Autodesk Inventor part; units mm, degrees
ref_plane "Work Plane3" through (10, 0, 0) normal (1, 0, 0) x (0, 1, 0)
ref_plane "Work Plane5" through (-12.5, 0, 0) normal (1, 0, 0) x (0, 1, 0)
ref_plane "XZ Plane" through (0, 0, 0) normal (0, 1, 0) x (-1, 0, 0)
sketch "Sketch19" plane through (0, 0, 0) normal (0, 0, 1) x (1, 0, 0)
  circle A0 centre (0, 0) radius 12.5
  dimension "d130" = 25
extrude "Extrusion17" add sketch "Sketch19" along normal blind 40
sketch "Sketch20" plane through (0, 0, 40) normal (0, 0, 1) x (1, 0, 0)
  circle A0 centre (0, 0) radius 10
  dimension "d133" = 20
fillet "Fillet6" radius 10 1 edges at (-12.5, 0, 0)
extrude "Extrusion18" cut sketch "Sketch20" against normal blind 36
ref_plane "Work Plane3" through (10, 0, 0) normal (1, 0, 0) x (0, 1, 0)
sketch "Sketch21" plane through (10, 0, 0) normal (1, 0, 0) x (0, 1, 0)
  line L0 (0, 0) -> (0, 20)
  circle A0 centre (0, 20) radius 2.85
  dimension "d138" = 20
  dimension "d139" = 5.7
extrude "Extrusion19" add sketch "Sketch21" along normal blind 14.5
sketch "Sketch26" plane through (0, 0, 0) normal (1, 0, 0) x (0, 1, 0)
  line L0 (-10, 40) -> (10, 40)
  line L1 (12.5, 40) -> (-12.5, 40)
  line L2 (10, 40) -> (12.5, 40)
  line L3 (17.5, 60) -> (12.5, 40)
  line L4 (17.5, 60) -> (17.5, 62.5)
  line L5 (17.5, 62.5) -> (15, 62.5)
  line L6 (15, 62.5) -> (15, 60)
  line L7 (10, 40) -> (15, 60)
  line L8 (0, -10.5) -> (0, 63)
  point P0 (0, 0)
  dimension "d147" = 2.5
  dimension "d148" = 2.5
revolve "Revolution1" add sketch "Sketch26" angle 360 about axis through (0, 0, -10) along (0, 0, 1)
sketch "Sketch27" plane through (0, 0, 0) normal (1, 0, 0) x (0, 1, 0)
  line L0 (12.5, 40) -> (13.7856, 41.5321)
  line L1 (12.5, 40) -> (14.5, 40) construction
  line L2 (13.7856, 41.5321) -> (17.5, 60)
  line L3 (12.5, 40) -> (-12.5, 40)
  line L4 (12.5, 40) -> (11.5, 40)
  line L5 (-17.5, 60) -> (17.5, 60)
  line L6 (17.5, 60) -> (16.5, 60)
  line L7 (16.5, 60) -> (11.5, 40)
  point P0 (0, 0)
  dimension "d150" = 2
  dimension "d151" = 50
  dimension "d152" = 1
  dimension "d153" = 1
extrude "Extrusion21" add sketch "Sketch27" along normal mid plane 2
pattern_circular "Circular Pattern2" count 8 over 360 about axis through (0, 0, -10) along (0, 0, 1) of "Extrusion21"
fillet "Fillet7" radius 5 1 edges at (-10, 0, 4)
ref_plane "Work Plane5" through (-12.5, 0, 0) normal (1, 0, 0) x (0, 1, 0)
sketch "Sketch30" plane through (-12.5, 0, 0) normal (1, 0, 0) x (0, 1, 0)
  circle A0 centre (0, 20) radius 2.85
  line L0 (0, 0) -> (0, 20)
  circle A1 centre (0, 20) radius 3.65
  line L1 (0, 20) -> (0, 35)
  circle A2 centre (0, 35) radius 2.15
  line L2 (0, 20) -> (-3.15, 20)
  line L3 (-3.15, 20) -> (3.15, 20)
  line L4 (2.15, 35) -> (3.15, 20)
  line L5 (-3.15, 20) -> (-2.1453, 35.1423)
  point P0 (2.9808, 20.3389)
  point P1 (-2.9809, 20.3376)
  point P2 (3.0126, 22.0607)
  point P3 (-3.0133, 22.0597)
  dimension "d166" = 7.3
  dimension "d167" = 15
  dimension "d168" = 4.3
  dimension "d169" = 3.15
  dimension "d170" = 6.3
extrude "Extrusion27" cut sketch "Sketch30" along normal blind 2
properties part number "Waterkanon poging 3" material "S235"
Work out the finished part from the listing and answer in its coordinate system (mm). A direction names the side the tool comes from. Give positions to 0.01 mm unless a question says otherwise; leave off trailing zeros. Loops run counter-clockwise (first coordinate to the right, second up) from the corner with the lowest first, then second, coordinate; pieces in that order, holes last. Notation, with made-up numbers: (57, -10) - (89, -10) arc R14 ccw to (89, -5) - close; hole circle Ø3 at (47, 89.5). An arc over 180 degrees is marked (long way). One line per question, with ' | ' between items.
(1) Each of these flat-tipped pins is pushed along its axis until it touches: pin 1 Ø12 at (x, z) = (13, 47.5) entering from +Y; pin 2 Ø5.5 at (x, z) = (14, 55) entering from +Y; pin 3 Ø4 at (x, y) = (3, -4.5) entering from -Z; pin 4 Ø5 at (x, y) = (-6.5, 12.5) entering from +Z. Where does it stop, or does it pass through?
Recorded:
pin 1: stops at y = 12.97 | pin 2: stops at y = 12.19 | pin 3: stops at z = 0.04 | pin 4: stops at z = 62.5
(2) A tool of negligible diameter and unlimited length cuts with its end or side. For faces 5 (the face through (-11.29, 0.11, 16.35)), 6 (the face through (18.249, 1.532, 17.597)), 7 (the face through (-14.8, -1, 47.8)), from which of +Z, -Z, +X, -X, +Y, -Y can it reach the whole face along a straight path? Write none if from no direction.
Recorded:
face 5: -X | face 6: +X | face 7: -Z, -X, -Y
(3) The mould has two halves that part along Y. Classify faces 1 (the face through (11.159, 9.745, 47.824)), 2 (the face through (-11.053, 11.033, 50.637)), 3 (the face through (0, 0, 4)), 4 (the face through (-1, -14.8, 47.8)): +Y half, -Y half, draft (parallel to the pull), parting line (faces both ways), or undercut.
Recorded:
face 1: undercut | face 2: +Y half | face 3: undercut | face 4: draft
(4) The part is cut by section B-B (z = 39). Write down the section's boundary in (x, y).
Recorded:
outline: circle Ø25 at (0, 0); hole circle Ø20 at (0, 0)
(5) Straight lines are drawn through the part: probe 1 along X at (y, z) = (0, 60.65); probe 2 along X at (y, z) = (5, 50.5). For each, find the intervals that lie inside material, in ascending order.
Recorded:
probe 1: x = -17.5 to -15, 15 to 17.5 | probe 2: x = -14.27 to -11.59, 11.59 to 14.27
(6) The part is cut by section A-A (z = 20). Write down the section's boundary in (x, y), then the cut area to 3 significant figures.
Recorded:
outline: (-11.96, -3.65) arc R12.5 ccw to (12.17, -2.85) - (24.5, -2.85) - (24.5, 2.85) - (12.17, 2.85) arc R12.5 ccw to (-11.96, 3.65) - (-10.5, 3.65) - (-10.5, -3.65) - close; hole circle Ø20 at (0, 0) | area: 232 mm²
